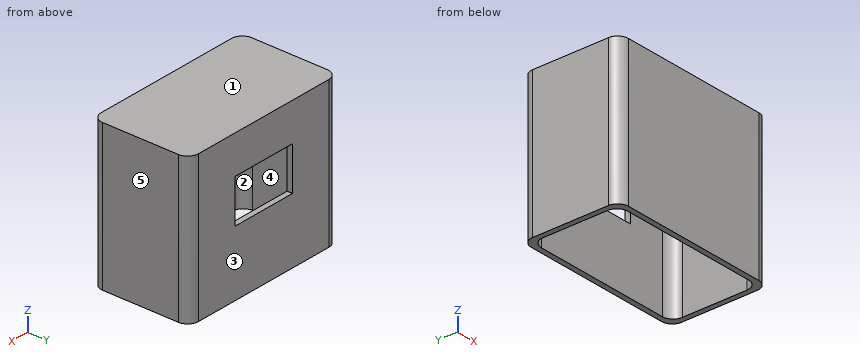
from build123d import *

# Parameters (mm, degrees)
BOSS_EXTRUDE1_DEPTH = 65
BOSS_EXTRUDE2_DEPTH = 2.5
CUT_EXTRUDE1_REACH  = 47
SKETCH4_W           = 31
SKETCH4_H           = 20


with BuildPart() as part:
    # Sketch2 → Boss-Extrude1 (new body)
    with BuildSketch(Plane.XY):
        with BuildLine():
            ThreePointArc((-40, 17.5), (-38.535533906, 21.035533906), (-35, 22.5))
            Line((-35, 22.5), (35, 22.5))
            ThreePointArc((35, 22.5), (38.535533906, 21.035533906), (40, 17.5))
            Line((40, 17.5), (40, -17.5))
            ThreePointArc((40, -17.5), (38.535533906, -21.035533906), (35, -22.5))
            Line((35, -22.5), (-35, -22.5))
            ThreePointArc((-35, -22.5), (-38.535533906, -21.035533906), (-40, -17.5))
            Line((-40, -17.5), (-40, 17.5))
        make_face()
        with BuildLine():
            ThreePointArc((-32.5, 20), (-36.035533906, 18.535533906), (-37.5, 15))
            Line((-37.5, 15), (-37.5, -15))
            ThreePointArc((-37.5, -15), (-36.035533906, -18.535533906), (-32.5, -20))
            Line((-32.5, -20), (32.5, -20))
            ThreePointArc((32.5, -20), (36.035533906, -18.535533906), (37.5, -15))
            Line((37.5, -15), (37.5, 15))
            ThreePointArc((37.5, 15), (36.035533906, 18.535533906), (32.5, 20))
            Line((32.5, 20), (-32.5, 20))
        make_face(mode=Mode.SUBTRACT)
    extrude(amount=BOSS_EXTRUDE1_DEPTH)

    # Sketch3 → Boss-Extrude2 (add)
    with BuildSketch(Plane.XY.offset(65)):
        with BuildLine():
            Line((-40, 17.5), (-40, -17.5))
            ThreePointArc((-40, -17.5), (-38.535533906, -21.035533906), (-35, -22.5))
            Line((-35, -22.5), (35, -22.5))
            ThreePointArc((35, -22.5), (38.535533906, -21.035533906), (40, -17.5))
            Line((40, -17.5), (40, 17.5))
            ThreePointArc((40, 17.5), (38.535533906, 21.035533906), (35, 22.5))
            Line((35, 22.5), (-35, 22.5))
            ThreePointArc((-35, 22.5), (-38.535533906, 21.035533906), (-40, 17.5))
        make_face()
    extrude(amount=BOSS_EXTRUDE2_DEPTH)

    # Sketch4 → Cut-Extrude1 (cut, up to next)
    with BuildSketch(Plane(origin=(0, 22.5, 0), x_dir=(1, 0, 0), z_dir=(0, 1, 0)), mode=Mode.PRIVATE) as cut_extrude1_sk1:
        with Locations((0, -40)):
            Rectangle(SKETCH4_W, SKETCH4_H)
    cut_extrude1_tool1 = extrude(cut_extrude1_sk1.sketch, amount=-CUT_EXTRUDE1_REACH, mode=Mode.PRIVATE) & part.part
    add(cut_extrude1_tool1.solids().sort_by_distance((0, 22.5, 40))[0], mode=Mode.SUBTRACT)


solid = part.part
Geometry: final body of the model. Coordinates: model frame, mm. Face numbers are marked on the shaded views. A direction names the side the tool comes from. Coordinates: 2 decimals unless noted, no trailing zeros. Loops run counter-clockwise (first coordinate to the right, second up) from the corner with the lowest first, then second, coordinate; pieces in that order, holes last. Notation, with made-up numbers: (14.25, 51) - (51.25, 51) arc R25 ccw to (51.25, 74) - close; hole circle Ø2 at (67, 33.25). An arc over 180 degrees is marked (long way). One line per question, with ' | ' between items. Start each with the question number.
(1) Draft query along Y for the marked faces 1, 2 and 3. Return one class per face: +Y half, -Y half, draft (parallel to the pull), parting line (faces both ways), or undercut.
(2) Reachability of the marked faces 4 and 5 from +Z, -Z, +X, -X, +Y, -Y: full face, straight path, thin tool, end or side. Return the list, or none.
(3) Cut plane C-C on y = 0. Output: boundary loops of the cut face in (x, z), and give its area (3 significant figures).
(4) Ray query, L1, parallel to Y at x = 12, z = 27.5; L2, parallel to X at y = 1, z = 23.5; L3, parallel to Z at x = 17, y = 0.5. Return the intervals inside material, ascending. Write a range as from..to.
(5) Cut plane A-A on x = -3.5. Output: boundary loops of the cut face in (y, z).
(6) First-contact query: pin 1 (3 mm diameter, centred on y = 21, z = 36, fed in from +X); pin 2 (2 mm diameter, centred on y = 21.5, z = 43, fed in from -X); pin 3 (5 mm diameter, centred on x = 15, y = -13, fed in from -Z). Flat tips, straight axial feed; report the tip coordinate or a pass-through.
(7) Cut plane D-D on z = 32.5. Output: boundary loops of the cut face in (x, y), and give its area (4 significant figures).
(8) Cut plane B-B on z = 62.5. Output: boundary loops of the cut face in (x, y).
Here are the results:
1) face 1: draft | face 2: undercut | face 3: +Y half
2) face 4: -Z | face 5: +Z, -Z, +X, +Y, -Y
3) outline: (-40, 0) - (-37.5, 0) - (-37.5, 65) - (37.5, 65) - (37.5, 0) - (40, 0) - (40, 67.5) - (-40, 67.5) - close | area: 525 mm²
4) L1: -22.5..-20, 20..22.5 | L2: -40..-37.5, 37.5..40 | L3: 65..67.5
5) outline: (-22.5, 0) - (-20, 0) - (-20, 65) - (20, 65) - (20, 50) - (22.5, 50) - (22.5, 67.5) - (-22.5, 67.5) - close; (20, 0) - (22.5, 0) - (22.5, 30) - (20, 30) - close
6) pin 1: x = 39.58 | pin 2: x = -39 | pin 3: z = 65
7) outline: (-40, -17.5) arc R5 ccw to (-35, -22.5) - (35, -22.5) arc R5 ccw to (40, -17.5) - (40, 17.5) arc R5 ccw to (35, 22.5) - (15.5, 22.5) - (15.5, 20) - (32.5, 20) arc R5 cw to (37.5, 15) - (37.5, -15) arc R5 cw to (32.5, -20) - (-32.5, -20) arc R5 cw to (-37.5, -15) - (-37.5, 15) arc R5 cw to (-32.5, 20) - (-15.5, 20) - (-15.5, 22.5) - (-35, 22.5) arc R5 ccw to (-40, 17.5) - close | area: 522.5 mm²
8) outline: (-40, -17.5) arc R5 ccw to (-35, -22.5) - (35, -22.5) arc R5 ccw to (40, -17.5) - (40, 17.5) arc R5 ccw to (35, 22.5) - (-35, 22.5) arc R5 ccw to (-40, 17.5) - close; hole (-37.5, -15) arc R5 ccw to (-32.5, -20) - (32.5, -20) arc R5 ccw to (37.5, -15) - (37.5, 15) arc R5 ccw to (32.5, 20) - (-32.5, 20) arc R5 ccw to (-37.5, 15) - close
